Autodesk Inventor part; units mm, degrees
ref_plane "YZ Plane" through (0, 0, 0) normal (1, 0, 0) x (0, 1, 0)
ref_plane "XZ Plane" through (0, 0, 0) normal (0, 1, 0) x (-1, 0, 0)
ref_plane "XY Plane" through (0, 0, 0) normal (0, 0, 1) x (1, 0, 0)
sketch "Sketch1" plane through (0, 0, 0) normal (0, 0, 1) x (1, 0, 0)
  line L0 (0, 0) -> (16, 0)
  line L1 (16, 0) -> (16, -10.16)
  line L2 (0, 0) -> (0, -20)
  arc A0 (0, -20) -> (5.3946, -14.6054) centre (0, -14.6054) ccw
  line L3 (0, -14.6054) -> (5.3946, -14.6054) construction
  line L4 (0, -14.6054) -> (0, -20) construction
  line L5 (5.3946, -14.6054) -> (16, -10.16)
  dimension "d0" = 16
  dimension "d1" = 20
  dimension "d2" = 10.16
  dimension "d3" = 90
  dimension "d4" = 5.3946
revolve "Revolution1" add sketch "Sketch1" angle 360 about axis through (0, 0, 0) along (0, -1, 0)
sketch "Sketch2" plane through (0, 0, 0) normal (0, 1, 0) x (1, 0, 0)
  circle A0 centre (0, 20.0361) radius 1.7
  circle A1 centre (0, -19.9639) radius 1.7
  line L0 (0, 24.0573) -> (0, -23.8232) construction
  line L1 (-3, 23.6661) -> (-3, 15.7162)
  line L2 (3, 23.6661) -> (3, 15.7162)
  line L3 (-3, 23.6661) -> (3, 23.6661)
  line L4 (-3, -23.5939) -> (-3, -15.7162)
  line L5 (3, -23.5939) -> (3, -15.7162)
  line L6 (-3, -23.5939) -> (3, -23.5939)
  circle A2 centre (0, 0) radius 16
  circle A3 centre (0, 0) radius 16
  dimension "d6" = 3.4
  dimension "d7" = 3.4
  dimension "d8" = 40
  dimension "d10" = 3
  dimension "d11" = 3
  dimension "d12" = 3.63
  dimension "d13" = 3
  dimension "d14" = 3
  dimension "d15" = 3.63
  dimension "d18" = 32
extrude "Extrusion1" add sketch "Sketch2" against normal blind 1.5875 contours L3 L2 A2 L1 | A2 L5 L6 L4
equation "\"d6\" = m3_clearance"
equation "\"d7\" = m3_clearance"
equation "\"d13\" = d11"
equation "\"d14\" = d13"
equation "\"d15\" = d12"
equation "\"m3_heat_set_insert\" = 4"
equation "\"m3_clearance\" = 3.4"
equation "\"m3_heat_set_depth\" = 7"
equation "\"robot_diameter\" = 354"
equation "\"hardboard_thickness\" = 5"
equation "\"motor_centerline_height\" = 13"
properties part number "ball_caster"
Check sheet for the modelled part. Datum: model origin and axes. Units: mm. A direction names the side the tool comes from. Coordinates: 2 decimals unless noted, no trailing zeros. Write each loop counter-clockwise with the first axis right and the second up, starting at its lowest first coordinate (ties: lowest second). Pieces come first, ordered by that corner, then holes. Notation, with made-up numbers: M -26,39.25 L -16,39.25 A23 cw -16,57.25 Z; hole C 2.5,-34.5 d3. An arc over 180 degrees is marked long. Write item = value, one per line. Start each with the question number.
1. Sectioned sample at D-D (y = -7.5). Record the cut outline in (x, z), then the cut area to 3 significant figures.
2. Tool access check on faces 1 (the flat face through (-3, -1, -20)), 2 (the flat face through (-3, -1, 20)), 3 (the flat face through (3, -1, -20)). Record the directions out of +Z, -Z, +X, -X, +Y, -Y that give a thin tool (end or side, any length) a straight path to the whole face; none if there is none.
3. Mould release check, pull along Z, two halves, no side actions. Record for faces 4 (the flat face through (-1.4, -1.588, 18.7)), 5 (the cylindrical face through (-3.47, -5.15, -15.62)), 6 (the cylindrical face through (-0.22, -0.78, -21.72)): pulls with the +Z half, pulls with the -Z half, needs draft (parallel to the pull), parting line crosses it, or undercut.
4. Sectioned sample at C-C (z = 0). Record the cut outline in (x, y).
5. Thickness scan on probe 1 along Z at (x, y) = (0, -1.1); probe 2 along X at (y, z) = (-2.5, -3); probe 3 along X at (y, z) = (-0.75, 22). Record the ranges inside material, lowest first.
6. Go/stop test with flat-tipped pins: pin 1 (4 mm diameter, centred on x = 0, z = 19.96, fed in from -Y); pin 2 (6 mm diameter, centred on y = -5, z = 6.5, fed in from +X); pin 3 (8 mm diameter, centred on x = 0, y = -13.5, fed in from +Z). Record where each tip stops, or that it passes through.
7. Sectioned sample at A-A (x = 0). Record the cut outline in (y, z).
8. Sectioned sample at B-B (z = 19). Record the cut outline in (x, y), then the cut area to 3 significant figures.
The answers:
q1.outline = C 0,0 d32
q1.area = 804 mm²
q2.face_1 = -Z, -X, +Y, -Y
q2.face_2 = +Z, -X, +Y, -Y
q2.face_3 = -Z, +X, +Y, -Y
q3.face_4 = needs draft
q3.face_5 = parting line crosses it
q3.face_6 = undercut
q4.outline = M -16,-10.16 L -5.39,-14.61 A5.39 ccw 5.39,-14.61 L 16,-10.16 L 16,0 L -16,0 Z
q5.probe_1 = -23.67 to -21.74, -18.34 to 18.26, 21.66 to 23.59
q5.probe_2 = -15.72 to 15.72
q5.probe_3 = -3 to 3
q6.pin_1 = -1.59
q6.pin_2 = 15.61
q6.pin_3 = 16
q7.outline = M -14.61,-5.39 L -10.16,-16 L -1.59,-16 L -1.59,-18.34 L 0,-18.34 L 0,18.26 L -1.59,18.26 L -1.59,16 L -10.16,16 L -14.61,5.39 A5.39 ccw Z; M -1.59,-23.67 L 0,-23.67 L 0,-21.74 L -1.59,-21.74 Z; M -1.59,21.66 L 0,21.66 L 0,23.59 L -1.59,23.59 Z
q8.outline = M -3,-1.59 L -1.4,-1.59 L -1.4,0 L -3,0 Z; M 1.4,-1.59 L 3,-1.59 L 3,0 L 1.4,0 Z
q8.area = 5.08 mm²
